The figure shows three views and two pictorial views of one solid part (mm, origin at its lowest corner). Answer the questions. Round coordinates to 2 decimals unless told otherwise and drop trailing zeros. Write each loop counter-clockwise with the first axis right and the second up, starting at its lowest first coordinate (ties: lowest second). Pieces come first, ordered by that corner, then holes. Notation, with made-up numbers: M 55.5,-24 L 95.5,-24 A16 cw 95.5,-10 Z; hole C 48.25,14 d6. An arc over 180 degrees is marked long. One line per item, written item: value. Start each with the question number.
Q1. Consider probe 1 along X at (y, z) = (119, 8.5); probe 2 along X at (y, z) = (50.5, 7.75); probe 3 along Y at (x, z) = (288.5, 7) (1 decimal). Determine where each line is inside the solid, lowest interval first.
Q2. Given pin 1 Ø1 at (x, z) = (157.5, 8) entering from -Y; pin 2 Ø3 at (x, z) = (176.5, 8.5) entering from -Y, each flat-ended and moving along its own axis, determine where each tip first touches the part or whether it passes through.
Q3. Find section B-B (y = 122). Write down the section's boundary in (x, z), and give its area (3 significant figures).
Q4. Find section A-A (z = 9.25). Write down the section's boundary in (x, y) (1 decimal), and give its area (3 significant figures).
Q5. Find section C-C (x = 225.5). Write down the section's boundary in (y, z) (1 decimal), and give its area (4 significant figures).
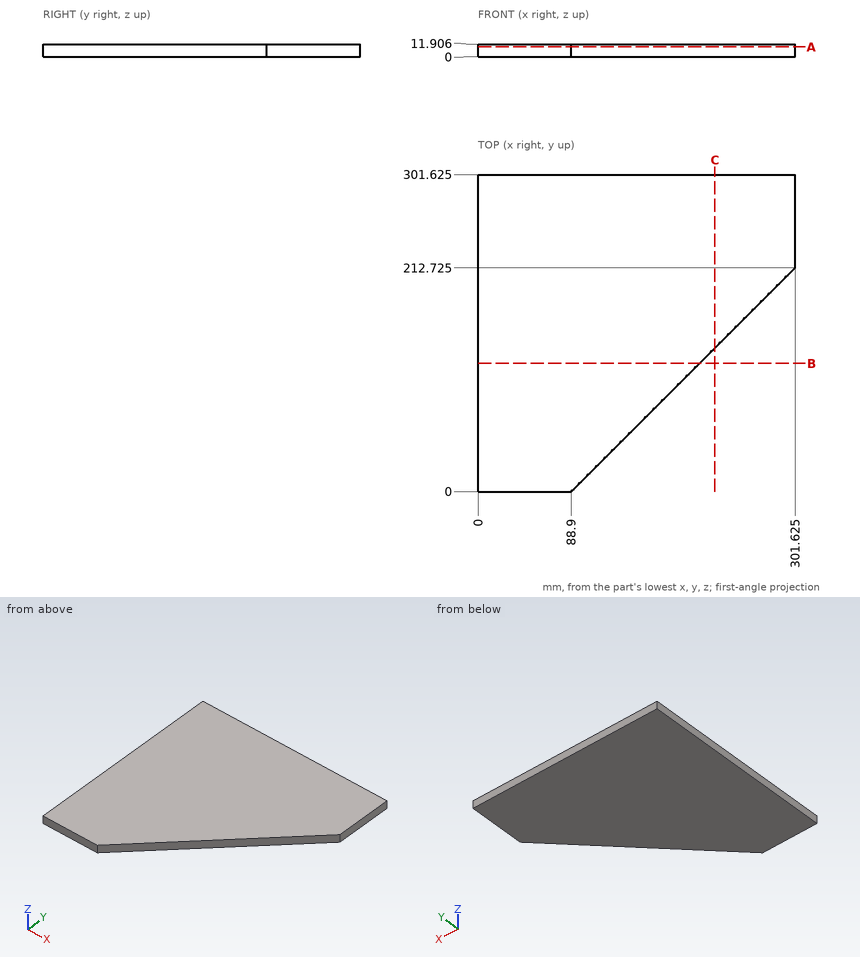
The answers:
1. probe 1: 0 to 207.9
1. probe 2: 0 to 139.4
1. probe 3: 199.6 to 301.6
2. pin 1: y = 68.1
2. pin 2: y = 86.1
3. outline: M 0,0 L 210.9,0 L 210.9,11.91 L 0,11.91 Z
3. area: 2,510 mm2
4. outline: M 0,0 L 88.9,0 L 301.6,212.7 L 301.6,301.6 L 0,301.6 Z
4. area: 68,400 mm2
5. outline: M 136.6,0 L 301.6,0 L 301.6,11.9 L 136.6,11.9 Z
5. area: 1,965 mm2
